```python
from build123d import *

# Parameters (mm, degrees)
SKETCH3_W           = 65
SKETCH3_H           = 65
BOSS_EXTRUDE2_DEPTH = 3
BOSS_EXTRUDE3_DEPTH = 65
CUT_EXTRUDE1_REACH  = 1619.511
SKETCH6_R           = 8
FILLET1_R           = 1


with BuildPart() as part:
    # Sketch3 → Boss-Extrude2 (new body)
    with BuildSketch(Plane.XZ.offset(-863.629465365)):
        with Locations((685.231990878, 1309.332866284)):
            Rectangle(SKETCH3_W, SKETCH3_H)
        with BuildLine():
            ThreePointArc((659.981990878, 1327.332866288), (660.3481074, 1326.448982809), (661.231990878, 1326.082866284))
            ThreePointArc((661.231990878, 1326.082866284), (662.115874352, 1326.448982806), (662.481990878, 1327.332866278))
            ThreePointArc((662.481990878, 1327.332866278), (662.115874357, 1328.216749759), (661.231990878, 1328.582866284))
            ThreePointArc((661.231990878, 1328.582866284), (660.348107403, 1328.216749762), (659.981990878, 1327.332866288))
        make_face(mode=Mode.SUBTRACT)
        with BuildLine():
            ThreePointArc((659.981990878, 1291.332866288), (660.3481074, 1290.448982809), (661.231990878, 1290.082866284))
            ThreePointArc((661.231990878, 1290.082866284), (662.115874352, 1290.448982806), (662.481990878, 1291.332866278))
            ThreePointArc((662.481990878, 1291.332866278), (662.115874357, 1292.216749759), (661.231990878, 1292.582866284))
            ThreePointArc((661.231990878, 1292.582866284), (660.348107403, 1292.216749762), (659.981990878, 1291.332866288))
        make_face(mode=Mode.SUBTRACT)
        with BuildLine():
            ThreePointArc((707.981990878, 1291.332866288), (708.3481074, 1290.448982809), (709.231990878, 1290.082866284))
            ThreePointArc((709.231990878, 1290.082866284), (710.115874352, 1290.448982806), (710.481990878, 1291.332866278))
            ThreePointArc((710.481990878, 1291.332866278), (710.115874357, 1292.216749759), (709.231990878, 1292.582866284))
            ThreePointArc((709.231990878, 1292.582866284), (708.348107403, 1292.216749762), (707.981990878, 1291.332866288))
        make_face(mode=Mode.SUBTRACT)
        with BuildLine():
            ThreePointArc((707.981990878, 1327.332866284), (708.348107402, 1326.448982808), (709.231990878, 1326.082866284))
            ThreePointArc((709.231990878, 1326.082866284), (710.115874352, 1326.448982805), (710.481990878, 1327.332866277))
            ThreePointArc((710.481990878, 1327.332866277), (710.115874357, 1328.216749758), (709.231990878, 1328.582866284))
            ThreePointArc((709.231990878, 1328.582866284), (708.348107402, 1328.216749761), (707.981990878, 1327.332866284))
        make_face(mode=Mode.SUBTRACT)
    extrude(amount=BOSS_EXTRUDE2_DEPTH)

    # Sketch4 → Boss-Extrude3 (add)
    with BuildSketch(Plane(origin=(0, 0, 1276.832866284), x_dir=(-1, 0, 0), z_dir=(0, 0, -1))):
        Polygon((-717.731990878, 860.629465365), (-717.731990878, 863.629465365), (-718.231990878, 863.629465365), (-718.231990878, 900.629465365), (-721.231990878, 900.629465365), (-721.231990878, 860.629465365), align=None)
    extrude(amount=-BOSS_EXTRUDE3_DEPTH)

    # Sketch6 → Cut-Extrude1 (cut, up to next)
    with BuildSketch(Plane(origin=(721.231990878, 0, 0), x_dir=(0, 0, -1), z_dir=(1, 0, 0)), mode=Mode.PRIVATE) as cut_extrude1_sk1:
        with Locations((-1309.332866284, 877.879465365)):
            Circle(SKETCH6_R)
    cut_extrude1_tool1 = extrude(cut_extrude1_sk1.sketch, amount=-CUT_EXTRUDE1_REACH, mode=Mode.PRIVATE) & part.part
    add(cut_extrude1_tool1.solids().sort_by_distance((721.231991, 877.879465, 1309.332866))[0], mode=Mode.SUBTRACT)

    # Fillet1
    fillet1_edges = [part.edges().sort_by_distance(p)[0] for p in [
        (718.231990878, 863.629465365, 1309.332866284),
    ]]
    fillet(fillet1_edges, radius=FILLET1_R)


solid = part.part
```
Build history of the part. All positions in model axes, mm. A direction names the side the tool comes from. Give positions to 0.01 mm unless a question says otherwise; leave off trailing zeros. Loops run counter-clockwise (first coordinate to the right, second up) from the corner with the lowest first, then second, coordinate; pieces in that order, holes last.
Item 1: Pull direction Y, two halves, no side cores. Call faces 3 (the face through (719.75, 873.01, 1315.68)), 4 (the face through (721.232, 880.9, 1301.7)), 5 (the face through (685, 863.629, 1309)): released by +Y, released by -Y, zero draft, split by the parting line, or undercut.
Answers follow:
face 3: undercut
face 4: zero draft
face 5: released by +Y
Item 2: Slice it at A-A, the plane z = 1316. List the corners of the cut face in (x, y).
Answers follow:
outline: (652.73, 860.63) - (721.23, 860.63) - (721.23, 873.46) - (718.23, 873.46) - (718.23, 864.63) arc R1 cw to (717.23, 863.63) - (652.73, 863.63) - close; (718.23, 882.3) - (721.23, 882.3) - (721.23, 900.63) - (718.23, 900.63) - close
Item 3: Slice it at D-D, the plane y = 866. List the corners of the cut face in (x, z).
Answers follow:
outline: (718.23, 1276.83) - (721.23, 1276.83) - (721.23, 1341.83) - (718.23, 1341.83) - close
Item 4: Slice it at B-B, the plane y = 877. List the corners of the cut face in (x, z), and give its area (3 significant figures).
Answers follow:
outline: (718.23, 1276.83) - (721.23, 1276.83) - (721.23, 1301.38) - (718.23, 1301.38) - close; (718.23, 1317.28) - (721.23, 1317.28) - (721.23, 1341.83) - (718.23, 1341.83) - close
area: 147 mm2
Item 5: Flat gauge pins, fed straight in: pin 1 (2 mm diameter, centred on x = 675.5, z = 1326, fed in from +Y); pin 2 (5 mm diameter, centred on x = 679, y = 867, fed in from -Z). Where does each tip first touch, or does it go through?
Answers follow:
pin 1: stops at y = 863.63
pin 2: passes through
Item 6: Drill centre lines: line 1 (X direction, y = 868, z = 1321.5); line 2 (Y direction, x = 668.5, z = 1315); line 3 (Y direction, x = 717.5, z = 1300). Where is each one in solid material? Low to high.
Answers follow:
line 1: x = 718.23 to 721.23
line 2: y = 860.63 to 863.63
line 3: y = 860.63 to 863.67
Item 7: Slice it at C-C, the plane z = 1304.5. List the corners of the cut face in (x, y).
Answers follow:
outline: (652.73, 860.63) - (721.23, 860.63) - (721.23, 871.5) - (718.23, 871.5) - (718.23, 864.63) arc R1 cw to (717.23, 863.63) - (652.73, 863.63) - close; (718.23, 884.25) - (721.23, 884.25) - (721.23, 900.63) - (718.23, 900.63) - close
Item 8: Which spindle directions (+Z, -Z, +X, -X, +Y, -Y) get a long thin tool onto all of the face, cutting with end or side? Do faces 1 (the face through (720, 900.629, 1309)), 2 (the face through (718.232, 886.4, 1308.9)). Say none if no direction does.
Answers follow:
face 1: +Z, -Z, +X, -X, +Y
face 2: +Z, -Z, -X, +Y
